from build123d import *

# Parameters (mm, degrees)
SKETCH1_W           = 387.35
SKETCH1_H           = 609.6
BOSS_EXTRUDE1_DEPTH = 6.35
SKETCH2_W           = 43.18
SKETCH2_H           = 135.128
CUT_EXTRUDE1_DEPTH  = 362.183288823
SKETCH4_W           = 25.4
SKETCH4_H           = 25.4
CUT_EXTRUDE3_DEPTH  = 362.183288823
FILLET1_R           = 2.54


with BuildPart() as part:
    # Sketch1 → Boss-Extrude1 (new body)
    with BuildSketch(Plane(origin=(0, 0, 0), x_dir=(1, 0, 0), z_dir=(0, 1, 0))):
        Rectangle(SKETCH1_W, SKETCH1_H)
    extrude(amount=BOSS_EXTRUDE1_DEPTH)

    # Sketch2 → Cut-Extrude1 (cut, through all)
    with BuildSketch(Plane(origin=(0, 6.35, 0), x_dir=(1, 0, 0), z_dir=(0, 1, 0))):
        with Locations((123.19, -195.8594)):
            Rectangle(SKETCH2_W, SKETCH2_H)
        with Locations((123.19, 110.236)):
            Rectangle(SKETCH2_W, SKETCH2_H)
        with Locations((-123.19, -195.8594)):
            Rectangle(SKETCH2_W, SKETCH2_H)
        with Locations((-123.19, 110.236)):
            Rectangle(SKETCH2_W, SKETCH2_H)
    extrude(amount=-CUT_EXTRUDE1_DEPTH, mode=Mode.SUBTRACT)

    # Sketch4 → Cut-Extrude3 (cut, through all)
    with BuildSketch(Plane(origin=(0, 0, 0), x_dir=(1, 0, 0), z_dir=(0, 1, 0))):
        with Locations((0, -12.7)):
            Rectangle(SKETCH4_W, SKETCH4_H)
    extrude(amount=CUT_EXTRUDE3_DEPTH, mode=Mode.SUBTRACT)

    # Fillet1
    fillet1_edges = [part.edges().sort_by_distance(p)[0] for p in [
        (-144.78, 3.175, -177.8),
        (-101.6, 3.175, -177.8),
    ]]
    fillet(fillet1_edges, radius=FILLET1_R)


solid = part.part
Geometry: final body of the model. Coordinates: model frame, mm. Coordinates: 2 decimals unless noted, no trailing zeros. Order: outer loops, then holes, each group sorted by start corner. A loop starts at its lowest first (then second) coordinate and runs counter-clockwise, first axis right, second up.
1) Section B-B (z = -52.5). Return loops of the section in (x, y) (3 decimals).
Result sheet:
outline: (-193.675, 0) - (-144.78, 0) - (-144.78, 6.35) - (-193.675, 6.35) - close; (-101.6, 0) - (101.6, 0) - (101.6, 6.35) - (-101.6, 6.35) - close; (144.78, 0) - (193.675, 0) - (193.675, 6.35) - (144.78, 6.35) - close
2) Ray query, probe 1 along Z at (x, y) = (102, 1.75); probe 2 along X at (y, z) = (4.25, -80.5) (3 decimals); probe 3 along Z at (x, y) = (1, 4). Return the intervals inside material, ascending.
Result sheet:
probe 1: z = -304.8 to -177.8, -42.67 to 128.3, 263.42 to 304.8
probe 2: x = -193.675 to -144.78, -101.6 to 101.6, 144.78 to 193.675
probe 3: z = -304.8 to 0, 25.4 to 304.8
3) Section A-A (y = 5). Return loops of the section in (x, z) (3 decimals).
Result sheet:
outline: (-193.675, -304.8) - (193.675, -304.8) - (193.675, 304.8) - (-193.675, 304.8) - close; hole (-144.78, -175.26) arc R2.54 ccw to (-142.24, -177.8) - (-104.14, -177.8) arc R2.54 ccw to (-101.6, -175.26) - (-101.6, -42.672) - (-144.78, -42.672) - close; hole (-144.78, 128.295) - (-101.6, 128.295) - (-101.6, 263.423) - (-144.78, 263.423) - close; hole (-12.7, 0) - (12.7, 0) - (12.7, 25.4) - (-12.7, 25.4) - close; hole (101.6, -177.8) - (144.78, -177.8) - (144.78, -42.672) - (101.6, -42.672) - close; hole (101.6, 128.295) - (144.78, 128.295) - (144.78, 263.423) - (101.6, 263.423) - close
